Part model, mm, in its own coordinate system. A direction names the side the tool comes from. Coordinates: 2 decimals unless noted, no trailing zeros. Order: outer loops, then holes, each group sorted by start corner. A loop starts at its lowest first (then second) coordinate and runs counter-clockwise, first axis right, second up.
```python
from build123d import *

# Parameters (mm, degrees)
ESQUISSE2_R             = 2
ENL_V_MAT_EXTRU_1_DEPTH = 32.06752542


with BuildPart() as part:
    # Esquisse1 → Révolution1 (revolve)
    with BuildSketch(Plane.XY, mode=Mode.PRIVATE) as r_volution1_sk:
        Polygon((0, 0), (5.5, 0), (5.5, 20), (4.5, 20), (4.5, 15), (-5.5, 15), (-5.5, 20.263157895), (-6.5, 20.263157895), (-6.5, 0), align=None)
    revolve(r_volution1_sk.sketch.rotate(Axis((-6.5, 0, 0), (1, 0, 0)), 90), axis=Axis((-6.5, 0, 0), (1, 0, 0)))

    # Esquisse2 → Enlèv. mat.-Extru.1 (cut, through all)
    with BuildSketch(Plane(origin=(5.5, 0, 0), x_dir=(0, 0, -1), z_dir=(1, 0, 0))):
        Circle(ESQUISSE2_R)
    extrude(amount=-ENL_V_MAT_EXTRU_1_DEPTH, mode=Mode.SUBTRACT)


solid = part.part
```
(1) Slice it at C-C, the plane x = -2.5. Give the cut face in (y, z), then the cut area to 3 significant figures.
(2) Tool access for faces 5 (the face through (4.5, -15, 3)), 6 (the face through (-6.01, 19.78, -4.39)), 7 (the face through (4.99, -0.88, -19.98)): list every direction of +Z, -Z, +X, -X, +Y, -Y with a clear straight run to the whole face (end or side of a thin tool).
(3) Drop flat-ended pins along their axis: pin 1 (3 mm diameter, centred on y = 0, z = 0, fed in from -X); pin 2 (2 mm diameter, centred on x = 0.5, y = 9, fed in from -Z); pin 3 (1.5 mm diameter, centred on x = 4, z = -12.5, fed in from -Y). Give the stop position or say it passes through.
(4) Slice it at D-D, the plane y = 16.5. Give the cut face in (x, z), then the cut area to 3 significant figures.
(5) Probe line 1 (Y direction, x = 1, z = 0); line 2 (X direction, y = -1, z = -15.5); line 3 (X direction, y = -14.5, z = -14). List the from-to ranges inside material, lowest first.
(6) Pull direction X, two halves, no side cores. Call faces 1 (the face through (5.5, 0, -4)), 2 (the face through (-6.5, 4, 0)), 3 (the face through (-5.5, -15, -3)), 4 (the face through (0, -2, 0)): +X half, -X half, draft (parallel to the pull), parting line (faces both ways), or undercut.
(7) Slice it at A-A, the plane z = 0. Give the cut face in (x, y).
Here are the results:
1. outline: circle Ø30 at (0, 0); hole circle Ø4 at (0, 0)
1. area: 694 mm2
2. face 5: none
2. face 6: +X, -X
2. face 7: +X
3. pin 1: passes through
3. pin 2: stops at z = -12.69
3. pin 3: stops at y = -16.04
4. outline: (-6.5, -11.76) - (-5.5, -11.76) - (-5.5, 11.76) - (-6.5, 11.76) - close; (4.5, -11.3) - (5.5, -11.3) - (5.5, 11.3) - (4.5, 11.3) - close
4. area: 46.1 mm2
5. line 1: y = -15 to -2, 2 to 15
5. line 2: x = -6.5 to -5.5, 4.5 to 5.5
5. line 3: x = -6.5 to -5.5
6. face 1: +X half
6. face 2: -X half
6. face 3: undercut
6. face 4: draft
7. outline: (-6.5, -20.26) - (-5.5, -20.26) - (-5.5, -15) - (4.5, -15) - (4.5, -20) - (5.5, -20) - (5.5, -2) - (-6.5, -2) - close; (-6.5, 2) - (5.5, 2) - (5.5, 20) - (4.5, 20) - (4.5, 15) - (-5.5, 15) - (-5.5, 20.26) - (-6.5, 20.26) - close
